Geometry check sheet. Reference: drawing and pictorial views, mm from the part's lowest x, y, z. Give positions to 0.01 mm unless a question says otherwise; leave off trailing zeros. Order: outer loops, then holes, each group sorted by start corner. A loop starts at its lowest first (then second) coordinate and runs counter-clockwise, first axis right, second up.
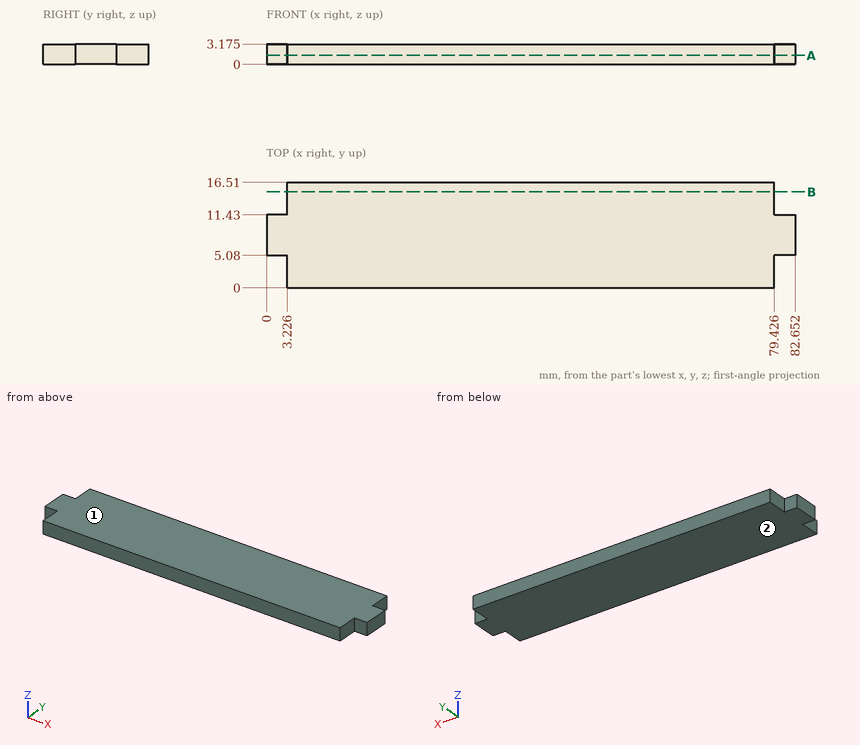
(1) Release check for a two-part mould opening along Z. For the marked faces 1 and 2 record: released by +Z, released by -Z, zero draft, split by the parting line, or undercut.
(2) Sectioned sample at B-B (y = 15). Enter the section's corners in (x, z) (1 decimal), plus the area to 3 significant figures.
(3) Sectioned sample at A-A (z = 1.4). Enter the section's corners in (x, y) (1 decimal).
(4) Thickness scan on L1, parallel to X at y = 14.75, z = 2.85 (1 decimal). Record the ranges inside material, lowest first.
(5) Go/stop test with flat-tipped pins: P1, Ø8, axis at x = 73.5, y = 5.5, coming from the -Z side; P2, Ø1.6, axis at x = 1, z = 1.5, coming from the -Y side; P3, Ø1.6, axis at y = 13.5, z = 1, coming from the -X side. Record where each tip stops, or that it passes through.
Values follow:
1. face 1: released by +Z
1. face 2: released by -Z
2. outline: (3.2, 0) - (79.4, 0) - (79.4, 3.2) - (3.2, 3.2) - close
2. area: 242 mm2
3. outline: (0, 5.1) - (3.2, 5.1) - (3.2, 0) - (79.4, 0) - (79.4, 5.1) - (82.7, 5.1) - (82.7, 11.4) - (79.4, 11.4) - (79.4, 16.5) - (3.2, 16.5) - (3.2, 11.4) - (0, 11.4) - close
4. L1: x = 3.2 to 79.4
5. P1: stops at z = 0
5. P2: stops at y = 5.08
5. P3: stops at x = 3.23
